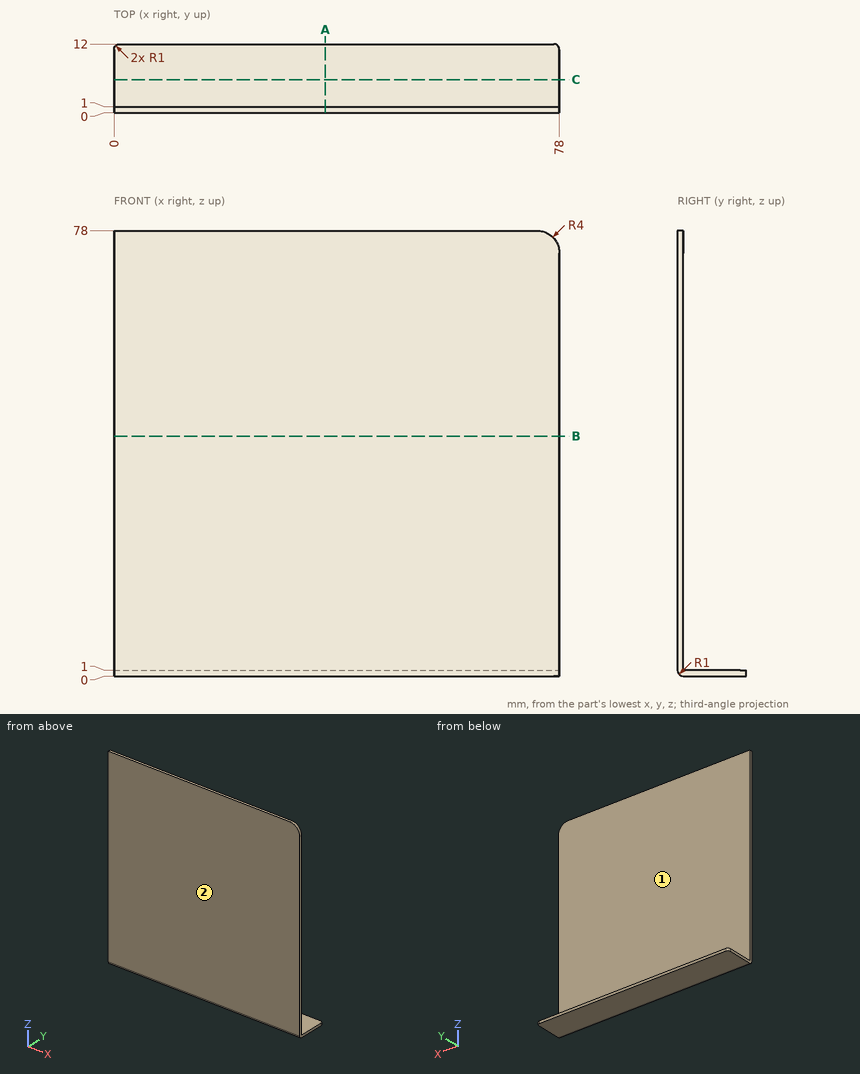
Answer from the drawing. Dimensions are ordinates in mm from the lowest x, y and z of the part. A direction names the side the tool comes from. Coordinates: 2 decimals unless noted, no trailing zeros. Write each loop counter-clockwise with the first axis right and the second up, starting at its lowest first coordinate (ties: lowest second). Pieces come first, ordered by that corner, then holes. Notation, with made-up numbers: M -16.75,-39.75 L -2.75,-39.75 A31 ccw -2.75,-11.75 Z; hole C -35,83.25 d10. An arc over 180 degrees is marked long. Use a Markdown table: item, result.
Q1. Which of the six approach directions +Z, -Z, +X, -X, +Y, -Y give full straight-line access (tool end or side, diameter ignored) to the marked faces 1 and 2?
Answer block:
| item | result |
|---|---|
| face 1 | +Z, +X, -X, +Y |
| face 2 | +Z, -Z, +X, -X, -Y |
Q2. The part is cut by section A-A, the plane x = 37. Write down the section's boundary in (y, z), then the cut area to 3 significant figures.
Answer block:
| item | result |
|---|---|
| outline | M 0,1 A1 ccw 1,0 L 12,0 L 12,1 L 1,1 L 1,78 L 0,78 Z |
| area | 88.8 mm2 |
Q3. This flat-tipped pin is pushed along its axis until it touches: pin 1 Ø8 at (x, z) = (11, 50) entering from +Y. Where does it stop, or does it pass through?
Answer block:
| item | result |
|---|---|
| pin 1 | stops at y = 1 |
Q4. A straight line is drawn through the part: L1, parallel to Y at x = 43, z = 43. Find the intervals that lie inside material, in ascending order. Write a range as [from, to].
Answer block:
| item | result |
|---|---|
| L1 | y = [0, 1] |
Q5. The part is cut by section B-B, the plane z = 42. Write down the section's boundary in (x, y).
Answer block:
| item | result |
|---|---|
| outline | M 0,0 L 78,0 L 78,1 L 0,1 Z |
